```python
from build123d import *

# Parameters (mm, degrees)
SKETCH_2_W      = 20
SKETCH_2_H      = 20
EXTRUDE_1_DEPTH = 2
CHAMFER_1_SIZE  = 1


with BuildPart() as part:
    # 스케치2 → 보스-돌출1 (new body)
    with BuildSketch(Plane.XY):
        Rectangle(SKETCH_2_W, SKETCH_2_H)
        Polygon((-3, -6.25), (-6.25, -6.25), (-6.25, 6.25), (-3, 6.25), (-3, 7.25), (-2, 7.25), (-2, 6.25), (2, 6.25), (2, 7.25), (3, 7.25), (3, 6.25), (6.25, 6.25), (6.25, -6.25), (3, -6.25), (3, -7.25), (2, -7.25), (2, -6.25), (-2, -6.25), (-2, -7.25), (-3, -7.25), align=None, mode=Mode.SUBTRACT)
    extrude(amount=EXTRUDE_1_DEPTH)

    # 모따기1
    chamfer_1_edges = [part.edges().sort_by_distance(p)[0] for p in [
        (6.25, -6.25, 1),
        (6.25, 6.25, 1),
        (-6.25, 6.25, 1),
        (-6.25, -6.25, 1),
    ]]
    chamfer(chamfer_1_edges, length=CHAMFER_1_SIZE)


solid = part.part
```
The model under review builds one solid part; all positions refer to its coordinate system, in mm. A direction names the side the tool comes from. Coordinates: 2 decimals unless noted, no trailing zeros. Write each loop counter-clockwise with the first axis right and the second up, starting at its lowest first coordinate (ties: lowest second). Pieces come first, ordered by that corner, then holes. Notation, with made-up numbers: (52.5, -2) -> (60.5, -2) arc R11 ccw to (60.5, 11) -> close; hole circle Ø5 at (-26, 65). An arc over 180 degrees is marked (long way). One line per item, written item: value. Start each with the question number.
Q1. The part is to be moulded in two halves that separate along Y. For faces 3 (the face through (-6.25, 0, 1)), 4 (the face through (-10, 0, 1)), 5 (the face through (0, 6.25, 1)), say which applies: +Y half, -Y half, draft (parallel to the pull), parting line (faces both ways), or undercut.
Q2. To check wall thickness, follow probe 1 along X at (y, z) = (6.75, 0.95); probe 2 along Y at (x, z) = (-0.75, 0.5). State the ranges of each line that lie inside material, in increasing order.
Q3. For faces 1 (the face through (2.5, 7.25, 1)), 2 (the face through (10, 0, 1)), list the 3-axis set-ups (+Z, -Z, +X, -X, +Y, -Y) from which the entire face can be reached by the end or side of a thin tool; tool diameter is ignored.
Q4. Add section C-C, the plane z = 0.4. Give the boundary of the cut face in (x, y).
Q5. Add section B-B, the plane y = -1.75. Give the boundary of the cut face in (x, z), then the cut area to 3 significant figures.
Q6. Add section A-A, the plane x = 2.25. Give the boundary of the cut face in (y, z), then the cut area to 3 significant figures.
Response:
1. face 3: undercut
1. face 4: draft
1. face 5: undercut
2. probe 1: -10 to -3, -2 to 2, 3 to 10
2. probe 2: -10 to -6.25, 6.25 to 10
3. face 1: +Z, -Z
3. face 2: +Z, -Z, +X, +Y, -Y
4. outline: (-10, -10) -> (10, -10) -> (10, 10) -> (-10, 10) -> close; hole (-6.25, -5.25) -> (-5.25, -6.25) -> (-3, -6.25) -> (-3, -7.25) -> (-2, -7.25) -> (-2, -6.25) -> (2, -6.25) -> (2, -7.25) -> (3, -7.25) -> (3, -6.25) -> (5.25, -6.25) -> (6.25, -5.25) -> (6.25, 5.25) -> (5.25, 6.25) -> (3, 6.25) -> (3, 7.25) -> (2, 7.25) -> (2, 6.25) -> (-2, 6.25) -> (-2, 7.25) -> (-3, 7.25) -> (-3, 6.25) -> (-5.25, 6.25) -> (-6.25, 5.25) -> close
5. outline: (-10, 0) -> (-6.25, 0) -> (-6.25, 2) -> (-10, 2) -> close; (6.25, 0) -> (10, 0) -> (10, 2) -> (6.25, 2) -> close
5. area: 15.0 mm²
6. outline: (-10, 0) -> (-7.25, 0) -> (-7.25, 2) -> (-10, 2) -> close; (7.25, 0) -> (10, 0) -> (10, 2) -> (7.25, 2) -> close
6. area: 11.0 mm²
